Input: part model. Units: mm. Frame: model coordinates. Face numbers are marked on the shaded views. A direction names the side the tool comes from. Coordinates: 2 decimals unless noted, no trailing zeros. Loops run counter-clockwise (first coordinate to the right, second up) from the corner with the lowest first, then second, coordinate; pieces in that order, holes last. Notation, with made-up numbers: (-6, 7.5) -> (41, 7.5) arc R8 ccw to (41, 11.5) -> close; hole circle Ø8 at (52.25, -17.75). An arc over 180 degrees is marked (long way). Put each result on its own line as item: value. Start each with the question number.
1) Set-up query: the marked faces 1, 2 and 3. Return all of +Z, -Z, +X, -X, +Y, -Y with unobstructed straight access to the full face (end or side cutting, diameter ignored); none if empty.
2) Cut plane A-A (y = 41). Return the cut outline in (x, z), plus the area to 3 significant figures.
3) Contact query for flat-ended pins moving along their axis: P1, Ø3, axis at x = -8.5, y = 69, coming from the -Z side; P2, Ø6.5, axis at y = 10, z = 26.83, coming from the +X side; P3, Ø4, axis at x = 2, y = 72, coming from the -Z side. Output: stop coordinate, or through.
4) Cut plane C-C (z = 17.5). Return the cut outline in (x, y).
5) Cut plane B-B (x = -39). Return the cut outline in (y, z).
6) Material intervals for L1, parallel to Y at x = -64.5, z = -4.5; L2, parallel to X at y = 71.5, z = 31; L3, parallel to Z at x = -15, y = 13.5, sorted ascending.
7) Pull-direction query (X, two-part tool) for the marked faces 4, 5 and 6; classes: pulls with the +X half, pulls with the -X half, needs draft (parallel to the pull), parting line crosses it, or undercut.
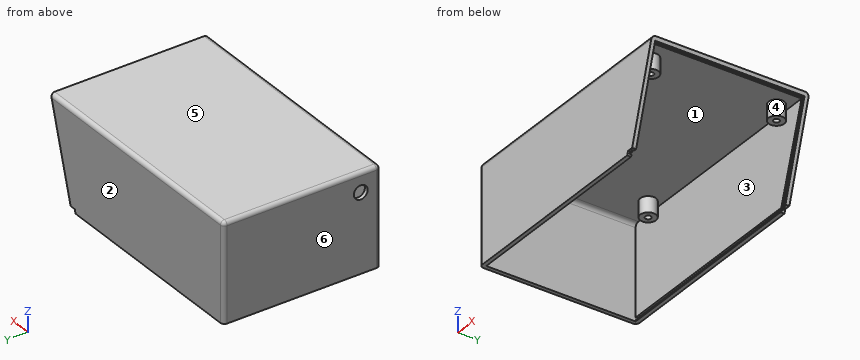
from build123d import *

# Parameters (mm, degrees)
BOSS_EXTRUDE1_DEPTH = 80
SHELL1_T            = -2
CUT_EXTRUDE2_DEPTH  = 92
CUT_EXTRUDE3_DEPTH  = 1
CUT_EXTRUDE4_DEPTH  = 1
SKETCH11_W          = 48.201532545
SKETCH11_H          = 76
CUT_EXTRUDE6_DEPTH  = 2
SKETCH12_W          = 2.088061302
SKETCH12_H          = 76
CUT_EXTRUDE7_DEPTH  = 2
CUT_EXTRUDE9_DEPTH  = 1
CUT_EXTRUDE10_DEPTH = 1
SKETCH16_R          = 3.5
CUT_EXTRUDE11_DEPTH = 2
SKETCH17_R          = 4
SKETCH17_R_2        = 1.5
BOSS_EXTRUDE2_DEPTH = 8
FILLET1_R           = 2


with BuildPart() as part:
    # Sketch2 → Boss-Extrude1 (new body)
    with BuildSketch(Plane(origin=(0, 0, 0), x_dir=(1, 0, 0), z_dir=(0, 1, 0))):
        Polygon((-108.645583258, -36.834647189), (-108.645583258, 13.165352811), (1.354416742, 13.165352811), (16.354416742, -36.834647189), align=None)
    extrude(amount=BOSS_EXTRUDE1_DEPTH)

    # Shell1
    shell1_openings = [part.faces().sort_by_distance(p)[0] for p in [
        (-53.645583258, 40, -13.165352811),
    ]]
    offset(amount=SHELL1_T, openings=shell1_openings, kind=Kind.INTERSECTION)

    # Sketch6 → Cut-Extrude2 (cut)
    with BuildSketch(Plane(origin=(0, 0, 0), x_dir=(-1, 0, 0), z_dir=(0, -1, 0))):
        Polygon((-1.354416742, 13.165352811), (-1.929112513, 11.24970024), (1.070887487, 11.24970024), (1.645583258, 13.165352811), align=None)
    extrude(amount=-CUT_EXTRUDE2_DEPTH, mode=Mode.SUBTRACT)

    # Sketch7 → Cut-Extrude3 (cut)
    with BuildSketch(Plane(origin=(0, 2, 0), x_dir=(1, 0, 0), z_dir=(0, 1, 0))):
        Polygon((-1.070887487, 11.24970024), (-106.645583258, 11.386355729), (-106.645583258, 12.207526526), (-1.358235373, 12.207526526), align=None)
    extrude(amount=-CUT_EXTRUDE3_DEPTH, mode=Mode.SUBTRACT)

    # Sketch9 → Cut-Extrude4 (cut)
    with BuildSketch(Plane(origin=(0, 78, 0), x_dir=(-1, 0, 0), z_dir=(0, -1, 0))):
        with BuildLine():
            Line((1.070887487, 11.24970024), (106.645583258, 11.208974605))
            ThreePointArc((106.645583258, 11.208974605), (106.645716747, 11.901071267), (106.645583258, 12.593167929))
            Line((106.645583258, 12.593167929), (1.358235373, 12.207526526))
            Line((1.358235373, 12.207526526), (1.070887487, 11.24970024))
        make_face()
    extrude(amount=-CUT_EXTRUDE4_DEPTH, mode=Mode.SUBTRACT)

    # Sketch11 → Cut-Extrude6 (cut)
    with BuildSketch(Plane(origin=(4.866075766, 0, -1.45982273), x_dir=(-0.287347886, 0, -0.957826285), z_dir=(0.957826285, 0, -0.287347886))):
        with Locations((-13.879834083, 40)):
            Rectangle(SKETCH11_W, SKETCH11_H)
    extrude(amount=-CUT_EXTRUDE6_DEPTH, mode=Mode.SUBTRACT)

    # Sketch12 → Cut-Extrude7 (cut)
    with BuildSketch(Plane(origin=(0, 0, -11.24970024), x_dir=(-1, 0, 0), z_dir=(0, 0, -1))):
        with Locations((-0.885081862, 40)):
            Rectangle(SKETCH12_W, SKETCH12_H)
    extrude(amount=-CUT_EXTRUDE7_DEPTH, mode=Mode.SUBTRACT)

    # Sketch14 → Cut-Extrude9 (cut)
    with BuildSketch(Plane(origin=(0, 2, 0), x_dir=(1, 0, 0), z_dir=(0, 1, 0))):
        Polygon((-1.070887487, 11.24970024), (0.429112513, 11.24970024), (14.821894685, -35.206342504), (13.8640684, -35.49369039), align=None)
    extrude(amount=-CUT_EXTRUDE9_DEPTH, mode=Mode.SUBTRACT)

    # Sketch15 → Cut-Extrude10 (cut)
    with BuildSketch(Plane(origin=(0, 78, 0), x_dir=(-1, 0, 0), z_dir=(0, -1, 0))):
        Polygon((-13.8640684, -35.49369039), (1.070887487, 11.24970024), (-0.429112513, 11.24970024), (-14.821894685, -35.206342504), align=None)
    extrude(amount=-CUT_EXTRUDE10_DEPTH, mode=Mode.SUBTRACT)

    # Sketch16 → Cut-Extrude11 (cut)
    with BuildSketch(Plane.ZY.offset(108.645583258)):
        with Locations((26.834647189, 10)):
            Circle(SKETCH16_R)
    extrude(amount=-CUT_EXTRUDE11_DEPTH, mode=Mode.SUBTRACT)

    # Sketch17 → Boss-Extrude2 (add)
    with BuildSketch(Plane(origin=(0, 0, 34.834647189), x_dir=(-1, 0, 0), z_dir=(0, 0, -1))):
        with Locations((89.1359316, 72.086299327)):
            Circle(SKETCH17_R)
        with Locations((89.1359316, 72.086299327)):
            Circle(SKETCH17_R_2, mode=Mode.SUBTRACT)
        with Locations((-3.8640684, 72.086299327)):
            Circle(SKETCH17_R)
        with Locations((-3.8640684, 72.086299327)):
            Circle(SKETCH17_R_2, mode=Mode.SUBTRACT)
        with Locations((-3.8640684, 8.086299327)):
            Circle(SKETCH17_R)
        with Locations((-3.8640684, 8.086299327)):
            Circle(SKETCH17_R_2, mode=Mode.SUBTRACT)
        with Locations((89.1359316, 8.086299327)):
            Circle(SKETCH17_R)
        with Locations((89.1359316, 8.086299327)):
            Circle(SKETCH17_R_2, mode=Mode.SUBTRACT)
    extrude(amount=BOSS_EXTRUDE2_DEPTH)

    # Fillet1
    fillet1_edges = [part.edges().sort_by_distance(p)[0] for p in [
        (-46.496042701, 2, 34.834647189),
        (-106.645583258, 40, 34.834647189),
        (-108.645583258, 80, 11.834647189),
        (-46.145583258, 80, 36.834647189),
        (-108.645583258, 0, 11.834647189),
        (-106.645583258, 2, 11.72414573),
        (-46.145583258, 0, 36.834647189),
        (-108.645583258, 40, 36.834647189),
    ]]
    fillet(fillet1_edges, radius=FILLET1_R)


solid = part.part
Results found:
1. face 1: -Z
1. face 2: +Z, -Z, +X, -X, +Y
1. face 3: -Z, +X
2. outline: (-108.65, -13.17) -> (-106.65, -13.17) -> (-106.65, 32.83) arc R2 cw to (-104.65, 34.83) -> (13.67, 34.83) -> (13.86, 35.49) -> (15.78, 34.92) -> (16.35, 36.83) -> (-106.65, 36.83) arc R2 ccw to (-108.65, 34.83) -> close
2. area: 345 mm2
3. P1: stops at z = 34.83
3. P2: stops at x = 7.86
3. P3: stops at z = 26.83
4. outline: (-108.65, 2) arc R2 ccw to (-106.65, 0) -> (10.55, 0) -> (10.55, 2) -> (9.34, 2) -> (9.34, 1) -> (8.11, 1) -> (8.11, 2) -> (-104.65, 2) arc R2 cw to (-106.65, 4) -> (-106.65, 78) -> (8.11, 78) -> (8.11, 79) -> (9.34, 79) -> (9.34, 78) -> (10.55, 78) -> (10.55, 80) -> (-106.65, 80) arc R2 ccw to (-108.65, 78) -> close
5. outline: (0, -13.17) -> (2, -13.17) -> (2, -12.21) -> (1, -12.21) -> (1, -11.3) -> (2, -11.3) -> (2, 32.83) arc R2 cw to (4, 34.83) -> (78, 34.83) -> (78, -11.24) -> (79, -11.24) -> (79, -12.35) -> (78, -12.35) -> (78, -13.17) -> (80, -13.17) -> (80, 34.83) arc R2 ccw to (78, 36.83) -> (2, 36.83) arc R2 ccw to (0, 34.83) -> close
6. L1: y = 0 to 2, 78 to 80
6. L2: x = -108.65 to -106.65, -93.09 to -90.52, -87.76 to -85.18, -0.09 to 2.48, 5.24 to 7.82
6. L3: z = 34.83 to 36.83
7. face 4: undercut
7. face 5: needs draft
7. face 6: pulls with the -X half
